from build123d import *

# Parameters (mm, degrees)
CYLINDER071_R             = 7
CYLINDER071_DEPTH         = 5
CYLINDER070_R             = 6
CYLINDER070_DEPTH         = 20
FUSION022_PLACEMENT_ANGLE = 90


with BuildPart() as cylinder071:
    # Cylinder071 → Cylinder071 (new body)
    with BuildSketch(Plane.XY):
        Circle(CYLINDER071_R)
    extrude(amount=CYLINDER071_DEPTH)


with BuildPart() as powerswitch001:
    # Cylinder070 → Cylinder070 (new body)
    with BuildSketch(Plane.XY):
        Circle(CYLINDER070_R)
    extrude(amount=CYLINDER070_DEPTH)

    # Fusion022: union Cylinder071
    add(cylinder071.part)


with BuildPart() as powerswitch001_1:
    # Fusion022 placement: moved
    add(powerswitch001.part.moved(Location((71, 7.5, 14))).rotate(Axis((71, 7.5, 14), (0, -1, 0)), FUSION022_PLACEMENT_ANGLE))


solid = powerswitch001_1.part
The model under review builds one solid part; all positions refer to its coordinate system, in mm. A direction names the side the tool comes from. Round coordinates to 2 decimals unless told otherwise and drop trailing zeros. Order: outer loops, then holes, each group sorted by start corner. A loop starts at its lowest first (then second) coordinate and runs counter-clockwise, first axis right, second up. Notation, with made-up numbers: (57, 14) -> (90, 14) arc R18 ccw to (90, 44) -> close; hole circle Ø11 at (64.25, 52). An arc over 180 degrees is marked (long way). Return JSON: item names as keys, results as strings.
1. For L1, parallel to X at y = 5, z = 7.5; L2, parallel to Z at x = 53.25, y = 11.5; L3, parallel to Z at x = 52.25, y = 12.5, list the stretches that pass through material, from the lowest coordinate up. Write a range as [from, to].
Answer block:
{"L1": "x = [66, 71]", "L2": "z = [9.53, 18.47]", "L3": "z = [10.68, 17.32]"}
2. For faces 1 (the face through (71, 8, 14)), 2 (the face through (58.605, 9.302, 19.723)), list the 3-axis set-ups (+Z, -Z, +X, -X, +Y, -Y) from which the entire face can be reached by the end or side of a thin tool; tool diameter is ignored.
Answer block:
{"face 1": "+Z, -Z, +X, +Y, -Y", "face 2": "-X"}
3. Take a section at D-D (x = 66.5). Write out the cut boundary in (y, z).
Answer block:
{"outline": "circle Ø14 at (7.5, 14)"}
4. Insertion check: P1, Ø1, axis at x = 64, y = 12, coming from the -Z side; P2, Ø1.5, axis at x = 67.5, y = 8.5, coming from the +Z side; P3, Ø5, axis at x = 68, y = 11.5, coming from the -Z side. Each pin has a flat end and moves straight along its axis. Give the tip position at first contact, or say it passes through.
Answer block:
{"P1": "stops at z = 9.53", "P2": "stops at z = 21", "P3": "stops at z = 7.16"}
5. Take a section at A-A (z = 14). Write out the cut boundary in (x, y).
Answer block:
{"outline": "(51, 1.5) -> (66, 1.5) -> (66, 0.5) -> (71, 0.5) -> (71, 14.5) -> (66, 14.5) -> (66, 13.5) -> (51, 13.5) -> close"}
6. Take a section at B-B (y = 7.5). Write out the cut boundary in (x, z).
Answer block:
{"outline": "(51, 8) -> (66, 8) -> (66, 7) -> (71, 7) -> (71, 21) -> (66, 21) -> (66, 20) -> (51, 20) -> close"}
7. Take a section at C-C (x = 62). Write out the cut boundary in (y, z), then the cut area to 3 significant figures.
Answer block:
{"outline": "circle Ø12 at (7.5, 14)", "area": "113 mm²"}
